```python
from build123d import *

# Parameters (mm, degrees)
SKETCH5_W               = 50.1536
SKETCH5_H               = 27.62
BOSS_EXTRUDE1_DEPTH     = 21
SKETCH6_R               = 5.2
CUT_EXTRUDE1_DEPTH      = 4
SKETCH7_R               = 4.95
CUT_EXTRUDE2_DEPTH      = 44.456728236
CUT_EXTRUDE3_START      = -3.048
SKETCH8_R               = 5.2
CUT_EXTRUDE3_DEPTH      = 3.048
SKETCH11_W              = 20.32
SKETCH11_H              = 6.1976
BOSS_EXTRUDE2_DEPTH     = 21
CUT_EXTRUDE4_DEPTH      = 52.113946521
CUT_EXTRUDE4_DEPTH_BACK = 52.113946521
SKETCH9_R               = 1.143
CUT_EXTRUDE5_START      = -15.2522
SKETCH12_W              = 13.208
SKETCH12_H              = 2.921
CUT_EXTRUDE5_DEPTH      = 15.2522
SKETCH13_R              = 4.9403
CUT_EXTRUDE6_DEPTH      = 8.89
SKETCH14_R              = 3.048
CUT_EXTRUDE7_DEPTH      = 6.35
CUT_EXTRUDE8_DEPTH      = 12.192
SKETCH16_R              = 7.6778
CUT_EXTRUDE9_DEPTH      = 1.778
SKETCH17_R              = 6.35
CUT_EXTRUDE10_DEPTH     = 44.23068691
SKETCH18_R              = 1.2
CUT_EXTRUDE11_DEPTH     = 43.689299066
SKETCH19_W              = 2.225
SKETCH19_H              = 21
BOSS_EXTRUDE3_DEPTH     = 23.89
SKETCH20_W              = 5.08
SKETCH20_H              = 9.90092
CUT_EXTRUDE12_DEPTH     = 46.986208701
CUT_EXTRUDE13_REACH     = 44.427
SKETCH23_W              = 8.89
SKETCH23_H              = 5.08
BOSS_EXTRUDE4_DEPTH     = 1.27
CUT_EXTRUDE15_DEPTH     = 6.35
CUT_EXTRUDE16_START     = -3.81
CUT_EXTRUDE16_DEPTH     = 3.81
SKETCH27_W              = 6.35
SKETCH27_H              = 7.62
BOSS_EXTRUDE6_DEPTH     = 7.62
CHAMFER1_SIZE           = 1.27
FILLET2_R               = 3.81
SKETCH28_W              = 3.81
SKETCH28_H              = 5.207
CUT_EXTRUDE17_DEPTH     = 5.08
SKETCH29_W              = 2.54
SKETCH29_H              = 5.08
CUT_EXTRUDE18_DEPTH     = 5.08
SKETCH30_R              = 1.7907
CUT_EXTRUDE19_DEPTH     = 43.599568856
SKETCH31_W              = 2.54
SKETCH31_H              = 1.62646495
CUT_EXTRUDE20_DEPTH     = 59.732256893
FILLET3_R               = 0.508
SKETCH32_R              = 2.5
CUT_EXTRUDE21_DEPTH     = 2.5
FILLET4_R               = 5.08
FILLET5_R               = 5.08
FILLET6_R               = 2.54
FILLET7_R               = 2.54
FILLET8_R               = 0.762
FILLET9_R               = 0.762


# Some blends are built 0.0001 mm under size
with BuildPart() as part:
    # Sketch5 → Boss-Extrude1 (new body)
    with BuildSketch(Plane.XY):
        with Locations((-12.4568, 0)):
            Rectangle(SKETCH5_W, SKETCH5_H)
    extrude(amount=BOSS_EXTRUDE1_DEPTH)

    # Sketch6 → Cut-Extrude1 (cut)
    with BuildSketch(Plane(origin=(0, 0, 0), x_dir=(-1, 0, 0), z_dir=(0, 0, -1))):
        Circle(SKETCH6_R)
    extrude(amount=-CUT_EXTRUDE1_DEPTH, mode=Mode.SUBTRACT)

    # Sketch7 → Cut-Extrude2 (cut, through all)
    with BuildSketch(Plane(origin=(0, 0, 4), x_dir=(-1, 0, 0), z_dir=(0, 0, -1))):
        Circle(SKETCH7_R)
    extrude(amount=-CUT_EXTRUDE2_DEPTH, mode=Mode.SUBTRACT)

    # Sketch8 → Cut-Extrude3 (cut)
    with BuildSketch(Plane.XY.offset(21).offset(CUT_EXTRUDE3_START)):
        with Locations(Location((0, 0, 0), (0, 0, 180))):
            Circle(SKETCH8_R)
    extrude(amount=CUT_EXTRUDE3_DEPTH, mode=Mode.SUBTRACT)

    # Sketch11 → Boss-Extrude2 (add)
    with BuildSketch(Plane(origin=(0, 0, 0), x_dir=(-1, 0, 0), z_dir=(0, 0, -1))):
        with Locations((-4.685, -13.1788)):
            Rectangle(SKETCH11_W, SKETCH11_H)
    extrude(amount=-BOSS_EXTRUDE2_DEPTH)

    # Sketch9 → Cut-Extrude4 (cut, two sides: drawn at the far end of the back side and taken through both)
    with BuildSketch(Plane.XZ.offset(13.81).offset(-CUT_EXTRUDE4_DEPTH_BACK)):
        with Locations(Location((4.685, 8.699, 0), (0, 0, 270))):
            Circle(SKETCH9_R)
    extrude(amount=CUT_EXTRUDE4_DEPTH + CUT_EXTRUDE4_DEPTH_BACK, mode=Mode.SUBTRACT)

    # Sketch12 → Cut-Extrude5 (cut)
    with BuildSketch(Plane(origin=(0, 0, 0), x_dir=(-1, 0, 0), z_dir=(0, 0, -1)).offset(CUT_EXTRUDE5_START)):
        with Locations((-4.685, -11.2738)):
            Rectangle(SKETCH12_W, SKETCH12_H)
    extrude(amount=CUT_EXTRUDE5_DEPTH, mode=Mode.SUBTRACT)

    # Sketch13 → Cut-Extrude6 (cut)
    with BuildSketch(Plane.XZ.offset(16.2776)):
        with Locations(Location((4.685, 8.699, 0), (0, 0, 270))):
            Circle(SKETCH13_R)
    extrude(amount=-CUT_EXTRUDE6_DEPTH, mode=Mode.SUBTRACT)

    # Sketch14 → Cut-Extrude7 (cut)
    with BuildSketch(Plane(origin=(0, 13.81, 0), x_dir=(1, 0, 0), z_dir=(0, 1, 0))):
        with Locations(Location((4.685, -8.699, 0), (0, 0, 180))):
            Circle(SKETCH14_R)
    extrude(amount=-CUT_EXTRUDE7_DEPTH, mode=Mode.SUBTRACT)

    # Sketch15 → Cut-Extrude8 (cut)
    with BuildSketch(Plane(origin=(0, 0, 0), x_dir=(-1, 0, 0), z_dir=(0, 0, -1))):
        Polygon((12.9286, 10.795), (12.9286, 13.81), (37.5336, 13.81), (37.5336, -13.81), (12.9286, -13.81), align=None)
    extrude(amount=-CUT_EXTRUDE8_DEPTH, mode=Mode.SUBTRACT)

    # Sketch16 → Cut-Extrude9 (cut)
    with BuildSketch(Plane(origin=(0, 0, 12.192), x_dir=(-1, 0, 0), z_dir=(0, 0, -1))):
        with Locations((23.7236, 0)):
            Circle(SKETCH16_R)
    extrude(amount=-CUT_EXTRUDE9_DEPTH, mode=Mode.SUBTRACT)

    # Sketch17 → Cut-Extrude10 (cut, through all)
    with BuildSketch(Plane(origin=(0, 0, 13.97), x_dir=(-1, 0, 0), z_dir=(0, 0, -1))):
        with Locations((23.7236, 0)):
            Circle(SKETCH17_R)
    extrude(amount=-CUT_EXTRUDE10_DEPTH, mode=Mode.SUBTRACT)

    # Sketch18 → Cut-Extrude11 (cut, through all)
    with BuildSketch(Plane(origin=(0, 0, 12.192), x_dir=(-1, 0, 0), z_dir=(0, 0, -1))):
        with Locations((15.7236, 8)):
            Circle(SKETCH18_R)
        with Locations((31.7236, 8)):
            Circle(SKETCH18_R)
        with Locations((31.7236, -8)):
            Circle(SKETCH18_R)
        with Locations((15.7236, -8)):
            Circle(SKETCH18_R)
    extrude(amount=-CUT_EXTRUDE11_DEPTH, mode=Mode.SUBTRACT)

    # Sketch19 → Boss-Extrude3 (add)
    with BuildSketch(Plane(origin=(0, -10.08, 0), x_dir=(1, 0, 0), z_dir=(0, 1, 0))):
        with Locations((13.7325, -10.5)):
            Rectangle(SKETCH19_W, SKETCH19_H)
    extrude(amount=BOSS_EXTRUDE3_DEPTH)

    # Sketch20 → Cut-Extrude12 (cut, through all)
    with BuildSketch(Plane(origin=(0, 0, 0), x_dir=(0, 0, -1), z_dir=(1, 0, 0))):
        with Locations((-8.699, 0)):
            Rectangle(SKETCH20_W, SKETCH20_H)
    extrude(amount=CUT_EXTRUDE12_DEPTH, mode=Mode.SUBTRACT)

    # Cut-Extrude13: up to this face of the body (flat: up to its plane)
    cut_extrude13_end = Plane(part.part.faces().sort_by_distance((9.310423436, 0, 6.159))[0])
    # Sketch22 → Cut-Extrude13 (cut, up to the picked face)
    with BuildSketch(Plane(origin=(0, 0, 11.239), x_dir=(-1, 0, 0), z_dir=(0, 0, -1)), mode=Mode.PRIVATE) as cut_extrude13_sk1:
        Polygon((0, 4.95046), (-17.421153116, 6.474613403), (-17.421153116, -6.474613403), (0, -4.95046), align=None)
    cut_extrude13_tool1 = split(extrude(cut_extrude13_sk1.sketch, amount=CUT_EXTRUDE13_REACH, mode=Mode.PRIVATE), bisect_by=cut_extrude13_end, keep=Keep.BOTH, mode=Mode.PRIVATE)
    add(cut_extrude13_tool1.solids().sort_by(Axis((9.097919, 0, 11.239), (0, 0, -1)))[0], mode=Mode.SUBTRACT)

    # Sketch23 → Boss-Extrude4 (add)
    with BuildSketch(Plane(origin=(14.845, 0, 0), x_dir=(0, 0, -1), z_dir=(1, 0, 0))):
        with Locations((-8.699, 11.27)):
            Rectangle(SKETCH23_W, SKETCH23_H)
    extrude(amount=BOSS_EXTRUDE4_DEPTH)

    # Sketch25 → Cut-Extrude15 (cut)
    with BuildSketch(Plane.XY.offset(11.239)):
        with BuildLine():
            Line((9.939, 2.754), (16.986034424, 2.754))
            Line((16.986034424, 2.754), (16.986034424, -2.754))
            Line((16.986034424, -2.754), (9.939, -2.754))
            ThreePointArc((9.939, -2.754), (7.185, 0), (9.939, 2.754))
        make_face()
    extrude(amount=CUT_EXTRUDE15_DEPTH, mode=Mode.SUBTRACT)

    # Sketch26 → Cut-Extrude16 (cut)
    with BuildSketch(Plane.XY.offset(6.159).offset(CUT_EXTRUDE16_START)):
        with BuildLine():
            Line((16.986034424, 2.754), (16.986034424, -2.754))
            Line((16.986034424, -2.754), (9.939, -2.754))
            ThreePointArc((9.939, -2.754), (7.185, 0), (9.939, 2.754))
            Line((9.939, 2.754), (16.986034424, 2.754))
        make_face()
    extrude(amount=CUT_EXTRUDE16_DEPTH, mode=Mode.SUBTRACT)

    # Sketch27 → Boss-Extrude6 (add)
    with BuildSketch(Plane(origin=(14.845, 0, 0), x_dir=(0, 0, -1), z_dir=(1, 0, 0))):
        with Locations((-8.699, -12.4676)):
            Rectangle(SKETCH27_W, SKETCH27_H)
    extrude(amount=BOSS_EXTRUDE6_DEPTH)

    # Chamfer1
    chamfer1_edges = [part.edges().sort_by_distance(p)[0] for p in [
        (14.845, 11.27, 13.144),
        (14.845, 11.27, 4.254),
        (14.845, 8.73, 8.699),
    ]]
    chamfer(chamfer1_edges, length=CHAMFER1_SIZE - 0.0001)  # a hair under: the kernel refuses the full size

    # Fillet2
    fillet2_edges = [part.edges().sort_by_distance(p)[0] for p in [
        (22.465, -16.2776, 8.699),
        (22.465, -8.6576, 8.699),
    ]]
    fillet(fillet2_edges, radius=FILLET2_R - 0.0001)  # a hair under: the kernel refuses the full size

    # Sketch28 → Cut-Extrude17 (cut)
    with BuildSketch(Plane(origin=(0, 13.81, 0), x_dir=(1, 0, 0), z_dir=(0, 1, 0))):
        with Locations((11.67, -8.699)):
            Rectangle(SKETCH28_W, SKETCH28_H)
    extrude(amount=-CUT_EXTRUDE17_DEPTH, mode=Mode.SUBTRACT)

    # Sketch29 → Cut-Extrude18 (cut)
    with BuildSketch(Plane.ZY.offset(-13.575)):
        with Locations((8.699, 11.27)):
            Rectangle(SKETCH29_W, SKETCH29_H)
    extrude(amount=-CUT_EXTRUDE18_DEPTH, mode=Mode.SUBTRACT)

    # Sketch30 → Cut-Extrude19 (cut, through all)
    with BuildSketch(Plane.XY.offset(11.874)):
        with Locations((18.655, -12.4676)):
            Circle(SKETCH30_R)
    extrude(amount=-CUT_EXTRUDE19_DEPTH, mode=Mode.SUBTRACT)

    # Sketch31 → Cut-Extrude20 (cut, through all)
    with BuildSketch(Plane(origin=(14.845, 0, 0), x_dir=(0, 0, -1), z_dir=(1, 0, 0))):
        with Locations((-8.699, 7.916767525)):
            Rectangle(SKETCH31_W, SKETCH31_H)
    extrude(amount=CUT_EXTRUDE20_DEPTH, mode=Mode.SUBTRACT)

    # Fillet3
    fillet3_edges = [part.edges().sort_by_distance(p)[0] for p in [
        (4.685, 7.46, 9.842),
    ]]
    fillet(fillet3_edges, radius=FILLET3_R)

    # Sketch32 → Cut-Extrude21 (cut)
    with BuildSketch(Plane.XY.offset(21)):
        with Locations((-15.7236, 8)):
            Circle(SKETCH32_R)
        with Locations((-31.7236, 8)):
            Circle(SKETCH32_R)
        with Locations((-31.7236, -8)):
            Circle(SKETCH32_R)
        with Locations((-15.7236, -8)):
            Circle(SKETCH32_R)
    extrude(amount=-CUT_EXTRUDE21_DEPTH, mode=Mode.SUBTRACT)

    # Fillet4
    fillet4_edges = [part.edges().sort_by_distance(p)[0] for p in [
        (-37.5336, -13.81, 16.596),
        (-37.5336, 13.81, 16.596),
    ]]
    fillet(fillet4_edges, radius=FILLET4_R)

    # Fillet5
    fillet5_edges = [part.edges().sort_by_distance(p)[0] for p in [
        (-12.9286, -13.81, 6.096),
        (-12.9286, 13.81, 6.096),
    ]]
    fillet(fillet5_edges, radius=FILLET5_R)

    # Fillet6
    fillet6_edges = [part.edges().sort_by_distance(p)[0] for p in [
        (14.845, 13.81, 1.49205),
        (14.845, -16.2776, 2.762),
        (14.845, 13.81, 17.70695),
        (14.845, -16.2776, 16.437),
    ]]
    fillet(fillet6_edges, radius=FILLET6_R)

    # Fillet7
    # the kernel refuses this fillet: 2.54 mm, written as the material it takes off along each edge
    with BuildSketch(Plane(origin=(-5.475, -16.2776, -6.34741987), x_dir=(1, 0, 0), z_dir=(0, 0, 1))) as fillet7_piece_1:
        with BuildLine():
            CenterArc((2.538967948, 2.54), FILLET7_R, 181.63337652, 88.36662348)
            Line((0, 2.4676), (-0.050779359, 2.466152))
            ThreePointArc((-0.050779359, 2.466152), (-0.0508, 1.2338), (-0.0508, 0))
            Line((-0.0508, 0), (0, -0.0508))
            Line((0, -0.0508), (2.538967948, -0.0508))
            Line((2.538967948, -0.0508), (2.538967948, 0))
        make_face()
    extrude(amount=33.694839739, mode=Mode.SUBTRACT)

    # Fillet8
    fillet8_edges = [part.edges().sort_by_distance(p)[0] for p in [
        (14.845, 6.24922921, 8.699),
        (14.845, -6.24922921, 8.699),
    ]]
    fillet(fillet8_edges, radius=FILLET8_R)

    # Fillet9
    fillet9_edges = [part.edges().sort_by_distance(p)[0] for p in [
        (14.845, -2.754, 14.414),
        (14.845, 2.754, 14.414),
        (14.845, 2.754, 4.254),
        (14.845, -2.754, 4.254),
    ]]
    fillet(fillet9_edges, radius=FILLET9_R)


solid = part.part
```
Input: part model. Units: mm. Frame: model coordinates. A direction names the side the tool comes from. Give positions to 0.01 mm unless a question says otherwise; leave off trailing zeros. Write item = value, one per line. Start each with the question number.
1) Cut plane A-A (y = 0). Give the number of separate pieces and of enclosed holes in the cut face, and give its area (3 significant figures).
2) Material intervals for L1, parallel to Z at x = 9.5, y = -4; L2, parallel to X at y = -3, z = 18 (3 decimals); L3, parallel to Y at x = 10.5, z = 10, sorted ascending. Write a range as [from, to].
3) Reachability of faces 5 (the face through (15.21, 11.33, 3.35)), 6 (the face through (7, 1, 11.239)), 7 (the face through (-4.96, -1.56, 19.45)), 8 (the face through (-11.48, -12.28, 6.18)), 9 (the face through (16.115, 11, 12)) from +Z, -Z, +X, -X, +Y, -Y: full face, straight path, thin tool, end or side. Return the list, or none.
4) Pin query (flat end, axial travel): pin 1 (3.5 mm diameter, centred on y = 12.5, z = 11, fed in from +X) (3 decimals); pin 2 (3 mm diameter, centred on x = 4.5, z = 9.5, fed in from -Y); pin 3 (2 mm diameter, centred on y = -3, z = 6.5, fed in from +X) (3 decimals). Return the tip coordinate at first contact, or that it passes through.
5) Draft query along Y for faces 1 (the face through (-17, -9, 18.5)), 2 (the face through (12, 11, 6.095)), 3 (the face through (14.081, 13.086, 18.393)), 4 (the face through (12, 2.754, 14)). Return one class per face: pulls with the +Y half, pulls with the -Y half, needs draft (parallel to the pull), parting line crosses it, or undercut.
Answers follow:
q1.separate_pieces = 4
q1.enclosed_holes = 0
q1.area = 344 mm^2
q2.L1 = [0, 6.16], [11.24, 21]
q2.L2 = [-37.534, -29.32], [-18.127, -4.247], [4.247, 14.845]
q2.L3 = [-16.28, -12.73], [-9.81, -5.87], [5.87, 8.73]
q3.face_5 = -Z, +X, +Y
q3.face_6 = +X
q3.face_7 = +Z
q3.face_8 = -Z, -X, -Y
q3.face_9 = +Z, -Z, +X, +Y
q4.pin_1 = 16.115
q4.pin_2 = -7.39
q4.pin_3 = 14.845
q5.face_1 = undercut
q5.face_2 = needs draft
q5.face_3 = pulls with the +Y half
q5.face_4 = undercut
